from build123d import *

# Parameters (mm, degrees)
SKETCH1_W           = 80
SKETCH1_H           = 25
SKETCH1_R           = 2
BOSS_EXTRUDE1_DEPTH = 1.5
SKETCH2_W           = 28.5
SKETCH2_H           = 1.5
BOSS_EXTRUDE2_DEPTH = 25
SKETCH3_R           = 1
CUT_EXTRUDE1_DEPTH  = 1.5


with BuildPart() as part:
    # Sketch1 → Boss-Extrude1 (new body)
    with BuildSketch(Plane(origin=(0, 0, 0), x_dir=(1, 0, 0), z_dir=(0, 1, 0))):
        Rectangle(SKETCH1_W, SKETCH1_H)
        with Locations((-25, 2.5)):
            Circle(SKETCH1_R, mode=Mode.SUBTRACT)
        with Locations((25, 2.5)):
            Circle(SKETCH1_R, mode=Mode.SUBTRACT)
    extrude(amount=BOSS_EXTRUDE1_DEPTH)

    # Sketch2 → Boss-Extrude2 (add)
    with BuildSketch(Plane(origin=(0, 1.5, 0), x_dir=(1, 0, 0), z_dir=(0, 1, 0))):
        with Locations((-25.75, 11.75)):
            Rectangle(SKETCH2_W, SKETCH2_H)
        with Locations((25.75, 11.75)):
            Rectangle(SKETCH2_W, SKETCH2_H)
    extrude(amount=BOSS_EXTRUDE2_DEPTH)

    # Sketch3 → Cut-Extrude1 (cut)
    with BuildSketch(Plane(origin=(0, 0, -12.5), x_dir=(-1, 0, 0), z_dir=(0, 0, -1))):
        with Locations((13.5, 7.5)):
            Circle(SKETCH3_R)
        with Locations((-13.5, 7.5)):
            Circle(SKETCH3_R)
    extrude(amount=-CUT_EXTRUDE1_DEPTH, mode=Mode.SUBTRACT)


solid = part.part
Part model, mm, in its own coordinate system. A direction names the side the tool comes from. Coordinates: 2 decimals unless noted, no trailing zeros. Write each loop counter-clockwise with the first axis right and the second up, starting at its lowest first coordinate (ties: lowest second). Pieces come first, ordered by that corner, then holes. Notation, with made-up numbers: (20.25, 23.5) - (63.25, 23.5) arc R29 ccw to (63.25, 56.5) - close; hole circle Ø3 at (-5.5, -38). An arc over 180 degrees is marked (long way). Put each result on its own line as item: value.
1. 3-axis set-ups, long thin cutter, end or side, ignore diameter. For faces 5 (the flat face through (26, 14, -11)), 6 (the flat face through (11.5, 14, -12)), 7 (the cylindrical face through (23.4, 0.7, -1.3)): which of +Z, -Z, +X, -X, +Y, -Y reach the whole face in a straight line?
Final values:
face 5: +Z, +X, -X, +Y
face 6: +Z, -Z, +Y
face 7: +Y, -Y
2. Probe line 1 along Y through (x, z) = (13.5, -11.65); line 2 along Y through (x, z) = (-8.5, -8.5); line 3 along Z through (x, y) = (-14.5, 12.75). List the from-to ranges inside material, lowest first. Write a range as [from, to].
Final values:
line 1: y = [0, 6.5], [8.5, 26.5]
line 2: y = [0, 1.5]
line 3: z = [-12.5, -11]
3. Band-saw the part on D-D (y = 7.5). Write the cut outline in (x, z), then the cut area to 3 significant figures.
Final values:
outline: (-40, -12.5) - (-14.5, -12.5) - (-14.5, -11) - (-40, -11) - close; (-12.5, -12.5) - (-11.5, -12.5) - (-11.5, -11) - (-12.5, -11) - close; (11.5, -12.5) - (12.5, -12.5) - (12.5, -11) - (11.5, -11) - close; (14.5, -12.5) - (40, -12.5) - (40, -11) - (14.5, -11) - close
area: 79.5 mm²
4. Band-saw the part on B-B (x = 13.5). Write the cut outline in (y, z).
Final values:
outline: (0, -12.5) - (6.5, -12.5) - (6.5, -11) - (1.5, -11) - (1.5, 12.5) - (0, 12.5) - close; (8.5, -12.5) - (26.5, -12.5) - (26.5, -11) - (8.5, -11) - close
5. Band-saw the part on C-C (z = -2.5). Write the cut outline in (x, y).
Final values:
outline: (-40, 0) - (-27, 0) - (-27, 1.5) - (-40, 1.5) - close; (-23, 0) - (23, 0) - (23, 1.5) - (-23, 1.5) - close; (27, 0) - (40, 0) - (40, 1.5) - (27, 1.5) - close
6. Band-saw the part on A-A (y = 3.5). Write the cut outline in (x, z).
Final values:
outline: (-40, -12.5) - (-11.5, -12.5) - (-11.5, -11) - (-40, -11) - close; (11.5, -12.5) - (40, -12.5) - (40, -11) - (11.5, -11) - close
7. Flat gauge pins, fed straight in: pin 1 Ø3 at (x, y) = (13.5, 7.5) entering from -Z; pin 2 Ø10 at (y, z) = (7, -1) entering from +X; pin 3 Ø6 at (x, z) = (18.5, -7.5) entering from +Y; pin 4 Ø12.5 at (x, y) = (20, 16) entering from +Z. Where does each tip first touch, or does it go through?
Final values:
pin 1: stops at z = -12.5
pin 2: passes through
pin 3: stops at y = 1.5
pin 4: stops at z = -11
8. Two-plate mould, pull along Z, no slides. Class faces 1 (the flat face through (26, 26.5, -12)), 2 (the flat face through (-1, 1, -12.5)), 3 (the flat face through (-1, 1, 12.5)), 4 (the cylindrical face through (-26.6, 0.7, -1.3)): +Z half, -Z half, draft (parallel to the pull), parting line (faces both ways), or undercut.
Final values:
face 1: draft
face 2: -Z half
face 3: +Z half
face 4: undercut
